Source: CAD feature listing. Evaluate the final solid. Frame: model axes, mm. A direction names the side the tool comes from. Round coordinates to 2 decimals unless told otherwise and drop trailing zeros. Loops run counter-clockwise (first coordinate to the right, second up) from the corner with the lowest first, then second, coordinate; pieces in that order, holes last.
(1) First-contact query: pin 1 Ø2.5 at (y, z) = (41.5, -1) entering from -X; pin 2 Ø4 at (y, z) = (43, 2) entering from +X; pin 3 Ø4 at (x, y) = (-42, -27.13) entering from +Z; pin 4 Ø2.5 at (x, y) = (-42, 35.37) entering from +Z. Flat tips, straight axial feed; report the tip coordinate or a pass-through.
(2) Material intervals for probe 1 along Y at (x, z) = (-42, -2.05); probe 2 along X at (y, z) = (-22, -2.5); probe 3 along X at (y, z) = (-41.5, 1.25), sorted ascending.
(3) Section B-B, the plane z = 2. Count the separate pieces of the cut face and the enclosed holes in it, plus the area to 3 significant figures.
(4) Mould query, pull axis Y, two halves, no side actions, for faces 4 (the flat face through (-34, 36.87, -1)), 5 (the flat face through (-39, -36.86, -1)), 6 (the flat face through (-43.7, -46, -0.2)), 7 (the flat face through (44, -43, 4)). Classes: pulls with the +Y half, pulls with the -Y half, needs draft (parallel to the pull), parting line crosses it, or undercut.
(5) Set-up query: faces 1 (the flat face through (40, 48, -1)), 2 (the flat face through (48, -40, -1)), 3 (the cylindrical face through (38.5, -27.1, -1.5)). Return all of +Z, -Z, +X, -X, +Y, -Y with unobstructed straight access to the full face (end or side cutting, diameter ignored); none if empty.
(6) Section A-A, the plane y = -27.13. Return the cut outline in (x, z), plus the area to 3 significant figures.
(7) Section C-C, the plane y = 27. Return the cut outline in (x, z).
Solid Edge part; units mm, degrees
sketch "Sketch1" plane through (0, 0, 0) normal (0, 0, 1) x (1, 0, 0)
  line L0 (-40, -50) -> (40, -50)
  line L1 (40, -50) -> (50, -50)
  line L2 (50, -50) -> (50, -40)
  line L3 (50, -40) -> (50, 40)
  line L4 (50, 50) -> (50, 40)
  line L5 (40, 50) -> (50, 50)
  line L6 (40, 50) -> (-40, 50)
  line L7 (-50, 50) -> (-40, 50)
  line L8 (-50, 40) -> (-50, 50)
  line L9 (-50, 40) -> (-50, -40)
  line L10 (-50, -40) -> (-50, -50)
  line L11 (-50, -50) -> (-40, -50)
extrude "Protrusion1" add sketch "Sketch1" against normal blind 5
sketch "Sketch2" plane through (0, 0, 0) normal (0, 0, 1) x (1, 0, 0)
  line L0 (50, 50) -> (40, 50)
  line L1 (40, 46) -> (40, 50)
  line L2 (40, 46) -> (46, 46)
  line L3 (46, 46) -> (46, 40)
  line L4 (46, 40) -> (50, 40)
  line L5 (50, 40) -> (50, 50)
  line L6 (50, -40) -> (50, -50)
  line L7 (50, -50) -> (40, -50)
  line L8 (40, -46) -> (40, -50)
  line L9 (46, -46) -> (40, -46)
  line L10 (46, -40) -> (46, -46)
  line L11 (46, -40) -> (50, -40)
  line L12 (-50, -50) -> (-40, -50)
  line L13 (-40, -46) -> (-40, -50)
  line L14 (-46, -46) -> (-40, -46)
  line L15 (-46, -40) -> (-46, -46)
  line L16 (-50, -40) -> (-46, -40)
  line L17 (-50, -40) -> (-50, -50)
  line L18 (-46, 40) -> (-46, 46)
  line L19 (-46, 46) -> (-40, 46)
  line L20 (-40, 46) -> (-40, 50)
  line L21 (-40, 50) -> (-50, 50)
  line L22 (-50, 50) -> (-50, 40)
  line L23 (-50, 40) -> (-46, 40)
  dimension "D1" = 40
  dimension "D2" = 40
  dimension "D3" = 50
  dimension "D4" = 50
  dimension "D5" = 50
  dimension "D6" = 50
  dimension "D7" = 40
  dimension "D8" = 46
  dimension "D9" = 46
  dimension "D10" = 50
  dimension "D11" = 50
  dimension "D12" = 40
  dimension "D13" = 50
  dimension "D14" = 50
  dimension "D15" = 50
  dimension "D16" = 40
extrude "ExtrudedCutout_1" cut sketch "Sketch2" against normal blind 11.3526
sketch "Sketch3" plane through (0, 0, 0) normal (0, 0, 1) x (1, 0, 0)
  circle A0 centre (-40, -42.86) radius 1.5
  circle A1 centre (-36.13, 42.87) radius 1.5
  circle A2 centre (40, -42.86) radius 1.5
  circle A3 centre (37.53, 42.87) radius 1.5
extrude "Cutout1" cut sketch "Sketch3" against normal blind 5
sketch "Sketch4" plane through (0, 0, 0) normal (0, 0, 1) x (0, 1, 0)
  line L0 (36.87, 44) -> (-36.86, 44)
  line L1 (-36.86, 44) -> (-36.86, 34)
  line L2 (-36.86, 34) -> (-44, 34)
  line L3 (-44, 34) -> (-44, -34)
  line L4 (-44, -34) -> (-36.86, -34)
  line L5 (-36.86, -34) -> (-36.86, -44)
  line L6 (-36.86, -44) -> (36.87, -44)
  line L7 (36.87, -44) -> (36.87, -31.53)
  line L8 (36.87, -31.53) -> (44, -31.53)
  line L9 (44, -31.53) -> (44, 30.13)
  line L10 (44, 30.13) -> (36.87, 30.13)
  line L11 (36.87, 30.13) -> (36.87, 44)
extrude "Cutout2" cut sketch "Sketch4" against normal blind 5
sketch "Sketch5" plane through (0, 0, 0) normal (0, 0, 1) x (1, 0, 0)
  line L0 (-46, 40) -> (-44, 40)
  line L1 (-44, 40) -> (-44, 46)
  line L2 (-44, 46) -> (-46, 46)
  line L3 (-46, 40) -> (-46, 46)
  line L4 (46, 46) -> (44, 46)
  line L5 (44, 46) -> (44, 40)
  line L6 (44, 40) -> (46, 40)
  line L7 (46, 40) -> (46, 46)
  line L8 (-46, -40) -> (-44, -40)
  line L9 (-44, -40) -> (-44, -46)
  line L10 (-44, -46) -> (-46, -46)
  line L11 (-46, -46) -> (-46, -40)
  line L12 (46, -46) -> (44, -46)
  line L13 (44, -46) -> (44, -40)
  line L14 (44, -40) -> (46, -40)
  line L15 (46, -40) -> (46, -46)
extrude "ExtrudedProtrusion_3" add sketch "Sketch5" along normal blind 5
sketch "Sketch6" plane through (-44, -43, 3) normal (1, 0, 0) x (0, 1, 0)
  circle A0 centre (0, -1) radius 1.5
  circle A1 centre (85.9991, -1) radius 1.5
extrude "ExtrudedCutout_14" cut sketch "Sketch6" against normal blind 2
sketch "Sketch7" plane through (44, 43, 2.5) normal (-1, 0, 0) x (0, -1, 0)
  circle A0 centre (0.0009, -0.5) radius 1.5
  circle A1 centre (86, -0.5) radius 1.5
extrude "ExtrudedCutout_15" cut sketch "Sketch7" against normal blind 2
fillet "Round_2" radius 1 8 edges at (45, 40, 5) (45, 46, 5) (-45, 40, 5) (-45, 46, 5) (-45, -46, 5) (-45, -40, 5) (45, -46, 5) (45, -40, 5)
sketch "Sketch8" plane through (0, 0, -5) normal (0, 0, -1) x (0, -1, 0)
  line L0 (-50, -50) -> (50, -50)
  line L1 (50, -50) -> (50, 50)
  line L2 (50, 50) -> (-50, 50)
  line L3 (-50, 50) -> (-50, -50)
  dimension "D1" = 50
  dimension "D2" = 50
extrude "ExtrudedCutout_16" cut sketch "Sketch8" against normal blind 2
sketch "Sketch9" plane through (0, 0, 0) normal (0, 0, 1) x (1, 0, 0)
  line L0 (-42, -23.63) -> (-44, -23.63)
  line L1 (-44, -23.63) -> (-44, -30.63)
  line L2 (-42, -30.63) -> (-44, -30.63)
  arc A0 (-42, -30.63) -> (-42, -23.63) centre (-42, -27.13) ccw
  line L3 (42, -23.63) -> (44, -23.63)
  line L4 (44, -30.63) -> (44, -23.63)
  line L5 (42, -30.63) -> (44, -30.63)
  arc A1 (42, -30.63) -> (42, -23.63) centre (42, -27.13) cw
  line L6 (42, 31.87) -> (44, 31.87)
  line L7 (44, 36.87) -> (44, 31.87)
  line L8 (38.5, 36.87) -> (44, 36.87)
  line L9 (38.5, 35.37) -> (38.5, 36.87)
  arc A2 (38.5, 35.37) -> (42, 31.87) centre (42, 35.37) ccw
  line L10 (-38.5, 35.37) -> (-38.5, 36.87)
  line L11 (-38.5, 36.87) -> (-44, 36.87)
  line L12 (-44, 36.87) -> (-44, 31.87)
  line L13 (-42, 31.87) -> (-44, 31.87)
  arc A3 (-42, 31.87) -> (-38.5, 35.37) centre (-42, 35.37) ccw
extrude "Protrusion2" add sketch "Sketch9" against normal blind 3
sketch "Sketch10" plane through (0, 0, 0) normal (0, 0, 1) x (1, 0, 0)
  circle A0 centre (-42, 35.37) radius 1.5
  circle A1 centre (42, 35.37) radius 1.5
  circle A2 centre (42, -27.13) radius 1.5
  circle A3 centre (-42, -27.13) radius 1.5
extrude "ExtrudedCutout_17" cut sketch "Sketch10" against normal blind 3
Output values:
1. pin 1: stops at x = -46
1. pin 2: stops at x = 46
1. pin 3: stops at z = 0
1. pin 4: passes through
2. probe 1: y = -46 to -36.86, -30.63 to -28.63, -25.63 to -23.63, 31.87 to 33.87, 36.87 to 46
2. probe 2: x = -50 to -44, 44 to 50
2. probe 3: x = -46 to -44, 44 to 46
3. separate pieces: 8
3. enclosed holes: 0
3. area: 24.0 mm2
4. face 4: undercut
4. face 5: undercut
4. face 6: pulls with the -Y half
4. face 7: needs draft
5. face 1: +Z, -Z, +X, +Y
5. face 2: +Z, -Z, +X, -Y
5. face 3: +Z, -Z
6. outline: (-50, -3) - (-43.5, -3) - (-43.5, 0) - (-50, 0) - close; (-40.5, -3) - (-38.5, -3) - (-38.5, 0) - (-40.5, 0) - close; (38.5, -3) - (40.5, -3) - (40.5, 0) - (38.5, 0) - close; (43.5, -3) - (50, -3) - (50, 0) - (43.5, 0) - close
6. area: 51.0 mm2
7. outline: (-50, -3) - (-44, -3) - (-44, 0) - (-50, 0) - close; (44, -3) - (50, -3) - (50, 0) - (44, 0) - close
